CAD build for the part. Positions are in the model's coordinates, mm. A direction names the side the tool comes from. Round coordinates to 2 decimals unless told otherwise and drop trailing zeros. Write each loop counter-clockwise with the first axis right and the second up, starting at its lowest first coordinate (ties: lowest second). Pieces come first, ordered by that corner, then holes. Notation, with made-up numbers: (71.5, 83.5) - (92.5, 83.5) arc R27 ccw to (92.5, 100.5) - close; hole circle Ø8 at (17.5, 76.25). An arc over 180 degrees is marked (long way). Use one line per item in the form item = value. Start each with the question number.
Item 1: Band-saw the part on A-A, the plane x = 9.5. List the corners of the cut face in (y, z).
Item 2: Band-saw the part on B-B, the plane y = 2.25. List the corners of the cut face in (x, z) (3 decimals).
Item 3: Band-saw the part on C-C, the plane z = 2.5. Give the number of separate pieces and of enclosed holes in the cut face, and give its area (3 significant figures).
Item 4: Pin check, flat tips, straight feed: pin 1 (5 mm diameter, centred on x = 15.5, z = -1.5, fed in from -Y); pin 2 (3 mm diameter, centred on x = 12.5, y = 5, fed in from -Z); pin 3 (1.8 mm diameter, centred on x = 13.45, y = 3.5, fed in from +Z); pin 4 (2 mm diameter, centred on y = 3, z = 0.5, fed in from +X). Stop position of each tip, or through.
Item 5: Drill centre lines: L1, parallel to Y at x = 9.5, z = 0.25; L2, parallel to Z at x = 3.5, y = 6.5; L3, parallel to Z at x = 17, y = 6.25. Where is each one in solid material? Low to high.
Item 6: Pull direction X, two halves, no side cores. Call faces 1 (the cylindrical face through (-6.497, 1.739, -0.196)), 2 (the flat face through (6.1, 2.5, 1.9)), 3 (the flat face through (5.06, 1.85, -4.45)), 4 (the flat face through (9, 0, 0)): +X half, -X half, draft (parallel to the pull), parting line (faces both ways), or undercut.
Item 7: Tool access for faces 5 (the flat face through (17.489, 3.451, 1.825)), 6 (the flat face through (6.1, 4.5, -1.9)), 7 (the cylindrical face through (4.54, 0.3, -4.45)): list every direction of +Z, -Z, +X, -X, +Y, -Y with a clear straight run to the whole face (end or side of a thin tool).
from build123d import *

# Parameters (mm, degrees)
SKETCH1_R           = 4.55
BOSS_EXTRUDE2_DEPTH = 7
CUT_EXTRUDE1_REACH  = 24.164
SKETCH3_R           = 1
FILLET4_R           = 1


with BuildPart() as part:
    # Sketch1 → Boss-Extrude2 (new body)
    with BuildSketch(Plane(origin=(0, 0, 0), x_dir=(1, 0, 0), z_dir=(0, 1, 0))):
        with BuildLine():
            Line((6.5, 3.5), (3.577981651, 5.426605505))
            ThreePointArc((3.577981651, 5.426605505), (-6.5, 0), (3.577981651, -5.426605505))
            Line((3.577981651, -5.426605505), (6.5, -3.5))
            Line((6.5, -3.5), (18.5, -3.5))
            Line((18.5, -3.5), (18.5, -1.655))
            Line((18.5, -1.655), (16.45, -2))
            Line((16.45, -2), (16.45, 2))
            Line((16.45, 2), (18.5, 1.655))
            Line((18.5, 1.655), (18.5, 3.5))
            Line((18.5, 3.5), (6.5, 3.5))
        make_face()
        with Locations(Location((0, 0, 0), (0, 0, 270))):
            Circle(SKETCH1_R, mode=Mode.SUBTRACT)
    extrude(amount=BOSS_EXTRUDE2_DEPTH)

    # Sketch2 → Cut-Revolve1 (revolve, cut)
    with BuildSketch(Plane(origin=(0, 0, 0), x_dir=(0, -1, 0), z_dir=(1, 0, 0))):
        with BuildLine():
            Line((-4.5, 6.805), (-4.5, 6.195))
            add(Edge.make_bspline(
                [(-4.5, 6.195), (-4.5, 5.595), (-3.5, 5.595), (-2.5, 5.595), (-2.5, 6.195)],
                knots=[0, 0, 0, 1.570796327, 1.570796327, 3.141592654, 3.141592654, 3.141592654], degree=2, weights=[1, 0.707106781, 1, 0.707106781, 1]))
            Line((-2.5, 6.195), (-2.5, 6.805))
            add(Edge.make_bspline(
                [(-2.5, 6.805), (-2.499999858, 7.405000085), (-3.5, 7.405000085), (-4.500000142, 7.405000085), (-4.5, 6.805)],
                knots=[3.141592512, 3.141592512, 3.141592512, 4.71238898, 4.71238898, 6.283185449, 6.283185449, 6.283185449], degree=2, weights=[1, 0.707106731, 1, 0.707106731, 1]))
        make_face()
    revolve(axis=Axis((0, 7.335318457, 0), (0, -1, 0)), mode=Mode.SUBTRACT)

    # Sketch3 → Cut-Extrude1 (cut, up to next)
    with BuildSketch(Plane.XY.offset(3.5), mode=Mode.PRIVATE) as cut_extrude1_sk1:
        with Locations((13.45, 3.5)):
            Circle(SKETCH3_R)
    cut_extrude1_tool1 = extrude(cut_extrude1_sk1.sketch, amount=-CUT_EXTRUDE1_REACH, mode=Mode.PRIVATE) & part.part
    # Sketch3 → Cut-Extrude1 (cut, up to next)
    with BuildSketch(Plane.XY.offset(3.5), mode=Mode.PRIVATE) as cut_extrude1_sk2:
        with Locations((9.5, 3.5)):
            Circle(SKETCH3_R)
    cut_extrude1_tool2 = extrude(cut_extrude1_sk2.sketch, amount=-CUT_EXTRUDE1_REACH, mode=Mode.PRIVATE) & part.part
    add(cut_extrude1_tool1.solids().sort_by_distance((13.45, 3.5, 3.5))[0], mode=Mode.SUBTRACT)
    add(cut_extrude1_tool2.solids().sort_by_distance((9.5, 3.5, 3.5))[0], mode=Mode.SUBTRACT)

    # Fillet4
    fillet4_edges = [part.edges().sort_by_distance(p)[0] for p in [
        (5.038990826, 7, -4.463302752),
        (5.038990826, 0, -4.463302752),
        (-6.5, 0, 0),
        (5.038990826, 0, 4.463302752),
        (5.038990826, 7, 4.463302752),
        (-6.5, 7, 0),
    ]]
    fillet(fillet4_edges, radius=FILLET4_R)


solid = part.part
Determined:
q1.outline = (0, -3.5) - (2.5, -3.5) - (2.5, 3.5) - (0, 3.5) - close; (4.5, -3.5) - (7, -3.5) - (7, 3.5) - (4.5, 3.5) - close
q2.outline = (3.578, -5.427) - (6.5, -3.5) - (18.5, -3.5) - (18.5, -1.655) - (16.45, -2) - (16.45, 2) - (18.5, 1.655) - (18.5, 3.5) - (6.5, 3.5) - (3.578, 5.427) arc R6.5 ccw (long way) to start; hole circle Ø9.1 at (0, 0)
q3.separate_pieces = 2
q3.enclosed_holes = 3
q3.area = 106 mm²
q4.pin_1 = 0
q4.pin_2 = -3.5
q4.pin_3 = through
q4.pin_4 = 16.45
q5.L1 = 0 to 2.5, 4.5 to 7
q5.L2 = -5.32 to -2.91, 2.91 to 5.32
q5.L3 = -3.5 to -1.91, 1.91 to 3.5
q6.face_1 = parting line
q6.face_2 = undercut
q6.face_3 = +X half
q6.face_4 = draft
q7.face_5 = +Y, -Y
q7.face_6 = none
q7.face_7 = -Z, +X, -Y
